from build123d import *

# Parameters (mm, degrees)
F0_W     = 50
F0_H     = 50
F1_DEPTH = 100


with BuildPart() as f1:
    # F0 (on Top) → F1 (new body)
    with BuildSketch(Plane.XY):
        Rectangle(F0_W, F0_H)
    extrude(amount=F1_DEPTH)

    # F2 (on Front) → F3 (revolve, cut)
    with BuildSketch(Plane.XZ):
        Polygon((0, 0), (1.5, 0), (1.5, 5), (6.5, 5), (6.5, 6.5), (15, 6.5), (15, 100), (0, 100), align=None)
    revolve(axis=Axis((0, 0, 50), (0, 0, -1)), mode=Mode.SUBTRACT)


solid = f1.part
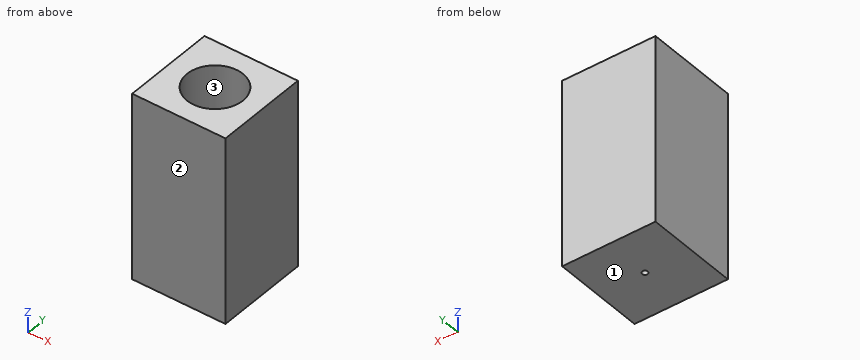
Could you check a few things on this model? Use its own coordinates, in mm. Face numbers are marked on the shaded views. Give positions to 0.01 mm unless a question says otherwise; leave off trailing zeros. Order: outer loops, then holes, each group sorted by start corner. A loop starts at its lowest first (then second) coordinate and runs counter-clockwise, first axis right, second up.
1. Suppose I cut it at B-B (z = 55.5). List the corners of the cut face in (x, y) for me.
2. I need wall thicknesses on L1, parallel to X at y = 0, z = 3.25; L2, parallel to X at y = 0, z = 79. Which ranges of each line are inside material? Lowest first, please.
3. Suppose I cut it at D-D (y = 9). List the corners of the cut face in (x, z) for me.
4. Suppose I cut it at A-A (x = 0). List the corners of the cut face in (y, z) for me, plus the area to 3 significant figures.
5. We'd pull the mould along Y, two halves only. Please class the marked faces 1, 2 and 3: pulls with the +Y half, pulls with the -Y half, needs draft (parallel to the pull), parting line crosses it, or undercut.
6. Will these pins go through, and if not, where does the flat tip stop? P1, Ø14.5, axis at x = 0.5, y = -1, coming from the +Z side; P2, Ø2, axis at x = -14, y = -6, coming from the -Z side.
Solved:
1. outline: (-25, -25) - (25, -25) - (25, 25) - (-25, 25) - close; hole circle Ø30 at (0, 0)
2. L1: x = -25 to -1.5, 1.5 to 25
2. L2: x = -25 to -15, 15 to 25
3. outline: (-25, 0) - (25, 0) - (25, 100) - (12, 100) - (12, 6.5) - (-12, 6.5) - (-12, 100) - (-25, 100) - close
4. outline: (-25, 0) - (-1.5, 0) - (-1.5, 5) - (-6.5, 5) - (-6.5, 6.5) - (-15, 6.5) - (-15, 100) - (-25, 100) - close; (1.5, 0) - (25, 0) - (25, 100) - (15, 100) - (15, 6.5) - (6.5, 6.5) - (6.5, 5) - (1.5, 5) - close
4. area: 2,160 mm2
5. face 1: needs draft
5. face 2: pulls with the -Y half
5. face 3: undercut
6. P1: stops at z = 6.5
6. P2: stops at z = 0
